```python
from build123d import *

# Parameters (mm, degrees)
F0_W     = 51.7186559737
F0_H     = 32.6044745743
F1_DEPTH = 10.16
F2_DEPTH = 15.494
F4_R     = 5.08
F5_R     = 5.07999
F6_DEPTH = 13.6398
F7_W     = 12.719899416
F7_H     = 10.316294618
F8_DEPTH = 1.7272


# Not quite as in the source:
# - a fillet or chamfer is up to 0.001 mm smaller than in the source, because OpenCascade refuses the exact size


with BuildPart() as f1:
    # F0 (on Top) → F1 (new body)
    with BuildSketch(Plane.XY):
        with Locations((25.8593279868, 16.3022372872)):
            Rectangle(F0_W, F0_H)
    extrude(amount=F1_DEPTH)

    # F2 (add): a face of the model
    f2_faces = [f1.faces().sort_by_distance(p)[0] for p in [
        (25.8593279868, 0, 5.08),
    ]]
    extrude(f2_faces, amount=F2_DEPTH)

    # F4
    f4_edges = [f1.edges().sort_by_distance(p)[0] for p in [
        (0, 8.555237, 10.16),
    ]]
    fillet(f4_edges, radius=F4_R)

    # F5 (radius 5.08 in the source; OpenCascade refuses exactly that, so slightly less here)
    f5_edges = [f1.edges().sort_by_distance(p)[0] for p in [
        (0, 8.555237, 0),
    ]]
    fillet(f5_edges, radius=F5_R)

    # F6 (add): a face of the model
    f6_faces = [f1.faces().sort_by_distance(p)[0] for p in [
        (26.3917193742, -15.494, 5.0799998568),
    ]]
    extrude(f6_faces, amount=F6_DEPTH)

    # F7 (on face) → F8 (join)
    with BuildSketch(Plane.XY.offset(10.16)):
        with Locations((30.7424403727, -16.3579261862)):
            Rectangle(F7_W, F7_H)
    extrude(amount=F8_DEPTH)


solid = f1.part
```
Part model, mm, in its own coordinate system. A direction names the side the tool comes from. Round coordinates to 2 decimals unless told otherwise and drop trailing zeros. Loops run counter-clockwise (first coordinate to the right, second up) from the corner with the lowest first, then second, coordinate; pieces in that order, holes last. Notation, with made-up numbers: (22.5, -33) -> (78.5, -33) arc R28 cw to (78.5, -3) -> close; hole circle Ø3 at (36.25, 4). An arc over 180 degrees is marked (long way). Use a Markdown table: item, result.
1) Cut at A-A, the plane x = 32. List the corners of the cut face in (y, z).
The answers:
| item | result |
|---|---|
| outline | (-29.13, 0) -> (32.6, 0) -> (32.6, 10.16) -> (-11.2, 10.16) -> (-11.2, 11.89) -> (-21.52, 11.89) -> (-21.52, 10.16) -> (-29.13, 10.16) -> close |
2) Cut at C-C, the plane z = 8.5. List the corners of the cut face in (x, y), and give its area (3 significant figures).
The answers:
| item | result |
|---|---|
| outline | (1.32, -29.13) -> (51.72, -29.13) -> (51.72, 32.6) -> (1.32, 32.6) -> close |
| area | 3,110 mm2 |
3) Drop flat-ended pins along their axis: pin 1 Ø6 at (y, z) = (24, 8.5) entering from -X; pin 2 Ø1.9 at (x, z) = (29.5, 11.5) entering from -Y; pin 3 Ø0.5 at (y, z) = (-14, 11) entering from +X. Give the stop position or say it passes through.
The answers:
| item | result |
|---|---|
| pin 1 | stops at x = 0.02 |
| pin 2 | stops at y = -21.52 |
| pin 3 | stops at x = 37.1 |
4) Probe line 1 (Z direction, x = 19.5, y = -26); line 2 (Y direction, x = 32.5, z = 10.5); line 3 (Z direction, x = 4.5, y = -10). List the from-to ranges inside material, lowest first. Write a range as [from, to].
The answers:
| item | result |
|---|---|
| line 1 | z = [0, 10.16] |
| line 2 | y = [-21.52, -11.2] |
| line 3 | z = [0.03, 10.13] |
5) Tool access for faces 1 (the flat face through (31, -16, 11.887)), 2 (the flat face through (31, -11.2, 11)), 3 (the flat face through (31, -21.516, 11)), 4 (the flat face through (24.382, -16, 11)), 5 (the flat face through (37.102, -16, 11)): list every direction of +Z, -Z, +X, -X, +Y, -Y with a clear straight run to the whole face (end or side of a thin tool).
The answers:
| item | result |
|---|---|
| face 1 | +Z, +X, -X, +Y, -Y |
| face 2 | +Z, +X, -X, +Y |
| face 3 | +Z, +X, -X, -Y |
| face 4 | +Z, -X, +Y, -Y |
| face 5 | +Z, +X, +Y, -Y |
